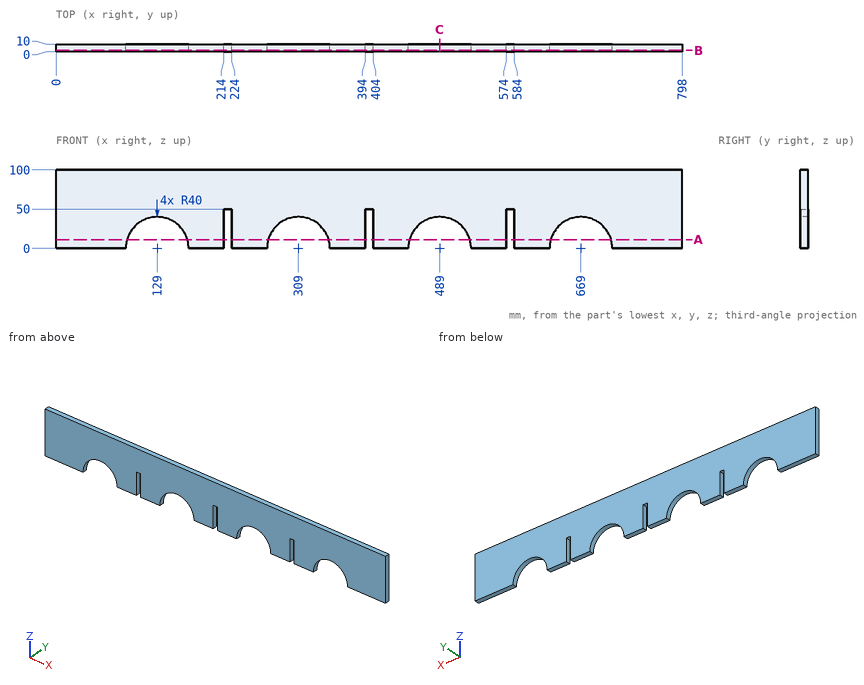
Check sheet for the drawn part. Datum: minimum x, y, z corner. Units: mm. Round coordinates to 2 decimals unless told otherwise and drop trailing zeros. Loops run counter-clockwise (first coordinate to the right, second up) from the corner with the lowest first, then second, coordinate; pieces in that order, holes last. Notation, with made-up numbers: (53, 34) - (67, 34) arc R19 ccw to (67, 59) - close; hole circle Ø2 at (22, -29.5). An arc over 180 degrees is marked (long way). Write item = value, one per line. Start each with the question number.
1. Section check A-A on z = 11. Give the number of separate pieces and of enclosed holes in the cut face, then the cut area to 3 significant figures.
2. Depth check by flat-ended pin: pin 1 (5 mm diameter, centred on x = 399, y = 2.5, fed in from -Z); pin 2 (2 mm diameter, centred on x = 492, y = 5, fed in from -Z). Enter the tip coordinate at first touch or a pass-through.
3. Section check B-B on y = 2. Enter the section's corners in (x, z), then the cut area to 3 significant figures.
4. Section check C-C on x = 489. Enter the section's corners in (y, z), then the cut area to 3 significant figures.
5. Thickness scan on line 1 (X direction, y = 2.5, z = 42.5); line 2 (Z direction, x = 686, y = 9); line 3 (Z direction, x = 461, y = 7). Record the ranges inside material, lowest first.
Working result:
q1.separate_pieces = 8
q1.enclosed_holes = 0
q1.area = 4,600 mm^2
q2.pin_1 = 50
q2.pin_2 = 39.8
q3.outline = (0, 0) - (89, 0) arc R40 cw to (169, 0) - (214, 0) - (214, 50) - (224, 50) - (224, 0) - (269, 0) arc R40 cw to (349, 0) - (394, 0) - (394, 50) - (404, 50) - (404, 0) - (449, 0) arc R40 cw to (529, 0) - (574, 0) - (574, 50) - (584, 50) - (584, 0) - (629, 0) arc R40 cw to (709, 0) - (798, 0) - (798, 100) - (0, 100) - close
q3.area = 68,200 mm^2
q4.outline = (0, 40) - (10, 40) - (10, 100) - (0, 100) - close
q4.area = 600 mm^2
q5.line_1 = 0 to 214, 224 to 394, 404 to 574, 584 to 798
q5.line_2 = 36.21 to 100
q5.line_3 = 28.57 to 100
